from build123d import *


with BuildPart() as part:
    # Esquisse1 → Révolution1 (revolve)
    with BuildSketch(Plane(origin=(0, 0, 0), x_dir=(1, 0, 0), z_dir=(0, 1, 0))):
        with BuildLine():
            Line((5.08, 4.7625), (4.7625, 4.445))
            Line((4.7625, 4.445), (4.7625, -4.445))
            Line((4.7625, -4.445), (5.08, -4.7625))
            Line((5.08, -4.7625), (7.3025, -4.7625))
            Line((7.3025, -4.7625), (7.553657425, -4.181328901))
            Line((7.553657425, -4.181328901), (7.952136973, -4.7625))
            Line((7.952136973, -4.7625), (11.224132695, -4.7625))
            Line((11.224132695, -4.7625), (12.438060247, -3.930171442))
            Line((12.438060247, -3.930171442), (12.772936813, -4.7625))
            Line((12.772936813, -4.7625), (13.49375, -4.7625))
            ThreePointArc((13.49375, -4.7625), (14.055016008, -4.530016008), (14.2875, -3.96875))
            Line((14.2875, -3.96875), (14.2875, 3.96875))
            ThreePointArc((14.2875, 3.96875), (14.055016008, 4.530016007), (13.49375, 4.7625))
            Line((13.49375, 4.7625), (12.772936813, 4.7625))
            Line((12.772936813, 4.7625), (12.438060247, 3.930171442))
            Line((12.438060247, 3.930171442), (11.224132694, 4.7625))
            Line((11.224132694, 4.7625), (7.952136973, 4.7625))
            Line((7.952136973, 4.7625), (7.553657425, 4.1813289))
            Line((7.553657425, 4.1813289), (7.3025, 4.7625))
            Line((7.3025, 4.7625), (5.08, 4.7625))
        make_face()
    revolve(axis=Axis((0, 0, -4.76375), (0, 0, 1)))


solid = part.part
CAD build for the part. Positions are in the model's coordinates, mm. Round coordinates to 2 decimals unless told otherwise and drop trailing zeros. Order: outer loops, then holes, each group sorted by start corner. A loop starts at its lowest first (then second) coordinate and runs counter-clockwise, first axis right, second up. Notation, with made-up numbers: (28.25, -4.75) - (48.25, -4.75) arc R17 cw to (48.25, 23.25) - close; hole circle Ø8 at (42, 49.5). An arc over 180 degrees is marked (long way). Return JSON: item names as keys, results as strings.
(1) Wall check: probe 1 along Y at (x, z) = (0, 1.25); probe 2 along X at (y, z) = (-1.75, -1.5). Give the ranges that are in metal, low to high. Write a range as from..to.
Answer key:
{"probe 1": "y = -14.29..-4.76, 4.76..14.29", "probe 2": "x = -14.18..-4.43, 4.43..14.18"}
(2) Pin check, flat tips, straight feed: pin 1 Ø1.5 at (y, z) = (-3, -3.5) entering from -X; pin 2 Ø2 at (x, z) = (-7.5, 3.5) entering from -Y. Stop position of each tip, or through.
Answer key:
{"pin 1": "stops at x = -14.11", "pin 2": "stops at y = -12.72"}
(3) Cut at A-A (z = -3.5). Give the cut face in (x, y) (1 decimal).
Answer key:
{"outline": "circle Ø28.6 at (0, 0); hole circle Ø9.5 at (0, 0)"}
(4) Pull direction Y, two halves, no side cores. Call faces 1 (the face through (-3.78, -2.9, 0.06)), 2 (the face through (-14.274, 0.628, -0.056)), 3 (the face through (5, -2, 4.763)): +Y half, -Y half, draft (parallel to the pull), parting line (faces both ways), or undercut.
Answer key:
{"face 1": "undercut", "face 2": "parting line", "face 3": "draft"}
